from build123d import *

# Parameters (mm, degrees)
F0_W     = 50
F0_H     = 17
F0_R     = 0.25
F0_R_2   = 0.5
F0_R_3   = 0.75
F0_R_4   = 1
F0_R_5   = 1.25
F0_R_6   = 1.5
F0_R_7   = 1.75
F0_R_8   = 2
F0_R_9   = 2.25
F0_R_10  = 2.5
F1_DEPTH = 3.5
F2_DEPTH = 7
F3_SIZE  = 2


with BuildPart() as f1:
    # F0 (on Top) → F1 (new body)
    with BuildSketch(Plane.XY):
        Rectangle(F0_W, F0_H)
        with Locations((-22.5, -3.75)):
            Circle(F0_R, mode=Mode.SUBTRACT)
        with Locations((-19.75, -3.75)):
            Circle(F0_R_2, mode=Mode.SUBTRACT)
        with Locations((-16.5, -3.75)):
            Circle(F0_R_3, mode=Mode.SUBTRACT)
        with Locations((-12.75, -3.75)):
            Circle(F0_R_4, mode=Mode.SUBTRACT)
        with Locations((-8.5, -3.75)):
            Circle(F0_R_5, mode=Mode.SUBTRACT)
        with Locations((-3.75, -3.75)):
            Circle(F0_R_6, mode=Mode.SUBTRACT)
        with Locations((1.5, -3.75)):
            Circle(F0_R_7, mode=Mode.SUBTRACT)
        with Locations((7.25, -3.75)):
            Circle(F0_R_8, mode=Mode.SUBTRACT)
        with Locations((13.5, -3.75)):
            Circle(F0_R_9, mode=Mode.SUBTRACT)
        with Locations((20.25, -3.75)):
            Circle(F0_R_10, mode=Mode.SUBTRACT)
        with Locations((-22.5, 3.75)):
            Circle(F0_R, mode=Mode.SUBTRACT)
        with Locations((-19.75, 3.75)):
            Circle(F0_R_2, mode=Mode.SUBTRACT)
        with Locations((-16.5, 3.75)):
            Circle(F0_R_3, mode=Mode.SUBTRACT)
        with Locations((-12.75, 3.75)):
            Circle(F0_R_4, mode=Mode.SUBTRACT)
        with Locations((-8.5, 3.75)):
            Circle(F0_R_5, mode=Mode.SUBTRACT)
        with Locations((-3.75, 3.75)):
            Circle(F0_R_6, mode=Mode.SUBTRACT)
        with Locations((1.5, 3.75)):
            Circle(F0_R_7, mode=Mode.SUBTRACT)
        with Locations((7.25, 3.75)):
            Circle(F0_R_8, mode=Mode.SUBTRACT)
        with Locations((13.5, 3.75)):
            Circle(F0_R_9, mode=Mode.SUBTRACT)
        with Locations((20.25, 3.75)):
            Circle(F0_R_10, mode=Mode.SUBTRACT)
    extrude(amount=F1_DEPTH)

    # F0 (on Top) → F2 (join, through all)
    with BuildSketch(Plane.XY):
        with Locations((-22.5, 3.75)):
            Circle(F0_R)
        with Locations((-19.75, 3.75)):
            Circle(F0_R_2)
        with Locations((-16.5, 3.75)):
            Circle(F0_R_3)
        with Locations((-12.75, 3.75)):
            Circle(F0_R_4)
        with Locations((-8.5, 3.75)):
            Circle(F0_R_5)
        with Locations((-3.75, 3.75)):
            Circle(F0_R_6)
        with Locations((1.5, 3.75)):
            Circle(F0_R_7)
        with Locations((7.25, 3.75)):
            Circle(F0_R_8)
        with Locations((13.5, 3.75)):
            Circle(F0_R_9)
        with Locations((20.25, 3.75)):
            Circle(F0_R_10)
    extrude(amount=F2_DEPTH)

    # F3
    f3_edges = [f1.edges().sort_by_distance(p)[0] for p in [
        (-25, -8.5, 1.75),
        (-25, 8.5, 1.75),
        (25, -8.5, 1.75),
        (25, 8.5, 1.75),
    ]]
    chamfer(f3_edges, length=F3_SIZE)


solid = f1.part
Part model, mm, in its own coordinate system. A direction names the side the tool comes from. Round coordinates to 2 decimals unless told otherwise and drop trailing zeros. Order: outer loops, then holes, each group sorted by start corner. A loop starts at its lowest first (then second) coordinate and runs counter-clockwise, first axis right, second up. Notation, with made-up numbers: (-7.5, -14.5) -> (22.5, -14.5) arc R22 cw to (22.5, -8.5) -> close; hole circle Ø1 at (29.25, -3). An arc over 180 degrees is marked (long way). Put each result on its own line as item: value.
Q1. Pin check, flat tip, straight feed: pin 1 Ø5 at (x, y) = (7.25, -3.75) entering from +Z. Stop position of the tip, or through.
From the geometry:
pin 1: stops at z = 3.5
Q2. Wall check: line 1 (Y direction, x = -19.75, z = 2.25); line 2 (Y direction, x = -3.75, z = 2.5); line 3 (Z direction, x = -22, y = -1.5). Give the ranges that are in metal, low to high. Write a range as [from, to].
From the geometry:
line 1: y = [-8.5, -4.25], [-3.25, 8.5]
line 2: y = [-8.5, -5.25], [-2.25, 8.5]
line 3: z = [0, 3.5]
Q3. Band-saw the part on D-D (y = -7). Give the cut face in (x, z).
From the geometry:
outline: (-24.5, 0) -> (24.5, 0) -> (24.5, 3.5) -> (-24.5, 3.5) -> close
Q4. Tool access for faces 5 (the face through (-24, 7.5, 1.7)), 6 (the face through (-2.32, 4.2, 5.23)): list every direction of +Z, -Z, +X, -X, +Y, -Y with a clear straight run to the whole face (end or side of a thin tool).
From the geometry:
face 5: +Z, -Z, -X, +Y
face 6: +Z
Q5. Band-saw the part on A-A (z = 5). State how many separate pieces and enclosed holes the cut face has, and give its area (3 significant figures).
From the geometry:
separate pieces: 10
enclosed holes: 0
area: 75.6 mm2
Q6. Band-saw the part on B-B (x = -3.75). Give the cut face in (y, z).
From the geometry:
outline: (-8.5, 0) -> (-5.25, 0) -> (-5.25, 3.5) -> (-8.5, 3.5) -> close; (-2.25, 0) -> (8.5, 0) -> (8.5, 3.5) -> (5.25, 3.5) -> (5.25, 7) -> (2.25, 7) -> (2.25, 3.5) -> (-2.25, 3.5) -> close
Q7. Pull direction Y, two halves, no side cores. Call faces 1 (the face through (-19.8, 3.8, 7)), 2 (the face through (-2.32, -3.3, 1.73)), 3 (the face through (5.252, -3.662, 1.726)), 4 (the face through (-13.487, 4.426, 5.226)): pulls with the +Y half, pulls with the -Y half, needs draft (parallel to the pull), parting line crosses it, or undercut.
From the geometry:
face 1: needs draft
face 2: undercut
face 3: undercut
face 4: parting line crosses it
